from build123d import *

# Parameters (mm, degrees)
SKETCH1_R             = 5.7
BOSS_EXTRUDE1_DEPTH   = 90
M8_TAPPED_HOLE1_D     = 6.8
M8_TAPPED_HOLE1_DEPTH = 35
M8_TAPPED_HOLE1_TIP   = 1.962990915
CHAMFER2_SIZE         = 1.5
SKETCH4_R             = 2.5
CUT_EXTRUDE1_DEPTH    = 10


with BuildPart() as part:
    # Sketch1 → Boss-Extrude1 (new body)
    with BuildSketch(Plane(origin=(0, 0, 0), x_dir=(1, 0, 0), z_dir=(0, 1, 0))):
        Circle(SKETCH1_R)
    extrude(amount=BOSS_EXTRUDE1_DEPTH)

    # M8 Tapped Hole1
    with Locations(Plane(origin=(0, 90, 0), x_dir=(1, 0, 0), z_dir=(0, 1, 0))):
        with Locations((0, 0)):
            Hole(M8_TAPPED_HOLE1_D / 2, depth=M8_TAPPED_HOLE1_DEPTH)
            with Locations((0, 0, -(M8_TAPPED_HOLE1_DEPTH + M8_TAPPED_HOLE1_TIP / 2))):  # 120° drill point
                Cone(0, M8_TAPPED_HOLE1_D / 2, M8_TAPPED_HOLE1_TIP, mode=Mode.SUBTRACT)

    # Chamfer2
    chamfer2_edges = [part.edges().sort_by_distance(p)[0] for p in [
        (-5.7, 0, 0),
        (-5.7, 90, 0),
    ]]
    chamfer(chamfer2_edges, length=CHAMFER2_SIZE)

    # Sketch4 → Cut-Extrude1 (cut, symmetric)
    with BuildSketch(Plane.XY):
        with Locations((0, 5)):
            Circle(SKETCH4_R)
    extrude(amount=CUT_EXTRUDE1_DEPTH, both=True, mode=Mode.SUBTRACT)


solid = part.part
Input: part model. Units: mm. Frame: model coordinates. Coordinates: 2 decimals unless noted, no trailing zeros. Order: outer loops, then holes, each group sorted by start corner. A loop starts at its lowest first (then second) coordinate and runs counter-clockwise, first axis right, second up.
1. Cut plane A-A, the plane y = 71.5. Return loops of the section in (x, z).
Checked values:
outline: circle Ø11.4 at (0, 0); hole circle Ø6.8 at (0, 0)
2. Contact query for flat-ended pins moving along their axis: P1, Ø3, axis at x = -2, z = 0.5, coming from the +Y side; P2, Ø6, axis at x = -4, y = 55, coming from the -Z side. Output: stop coordinate, or through.
Checked values:
P1: stops at y = 90
P2: stops at z = -5.61
3. Draft query along Y for faces 1 (the flat face through (2, 90, 3)), 2 (the cylindrical face through (0.74, 72.26, 3.32)), 3 (the cylindrical face through (2.385, 5.751, 0.08)), 4 (the flat face through (0, 0, 0)). Return one class per face: +Y half, -Y half, draft (parallel to the pull), parting line (faces both ways), or undercut.
Checked values:
face 1: +Y half
face 2: draft
face 3: undercut
face 4: -Y half
4. Cut plane B-B, the plane y = 5. Return loops of the section in (x, z).
Checked values:
outline: (-2.5, -5.12) - (-2.5, 5.12) arc R5.7 ccw to start; (2.5, -5.12) arc R5.7 ccw to (2.5, 5.12) - close
5. Cut plane C-C, the plane y = 34.5. Return loops of the section in (x, z).
Checked values:
outline: circle Ø11.4 at (0, 0)
6. Ray query, line 1 along Z through (x, y) = (-0.25, 74.5); line 2 along Y through (x, z) = (0, -3.25). Return the intervals inside material, ascending.
Checked values:
line 1: z = -5.69 to -3.39, 3.39 to 5.69
line 2: y = 0 to 2.5, 7.5 to 54.91
